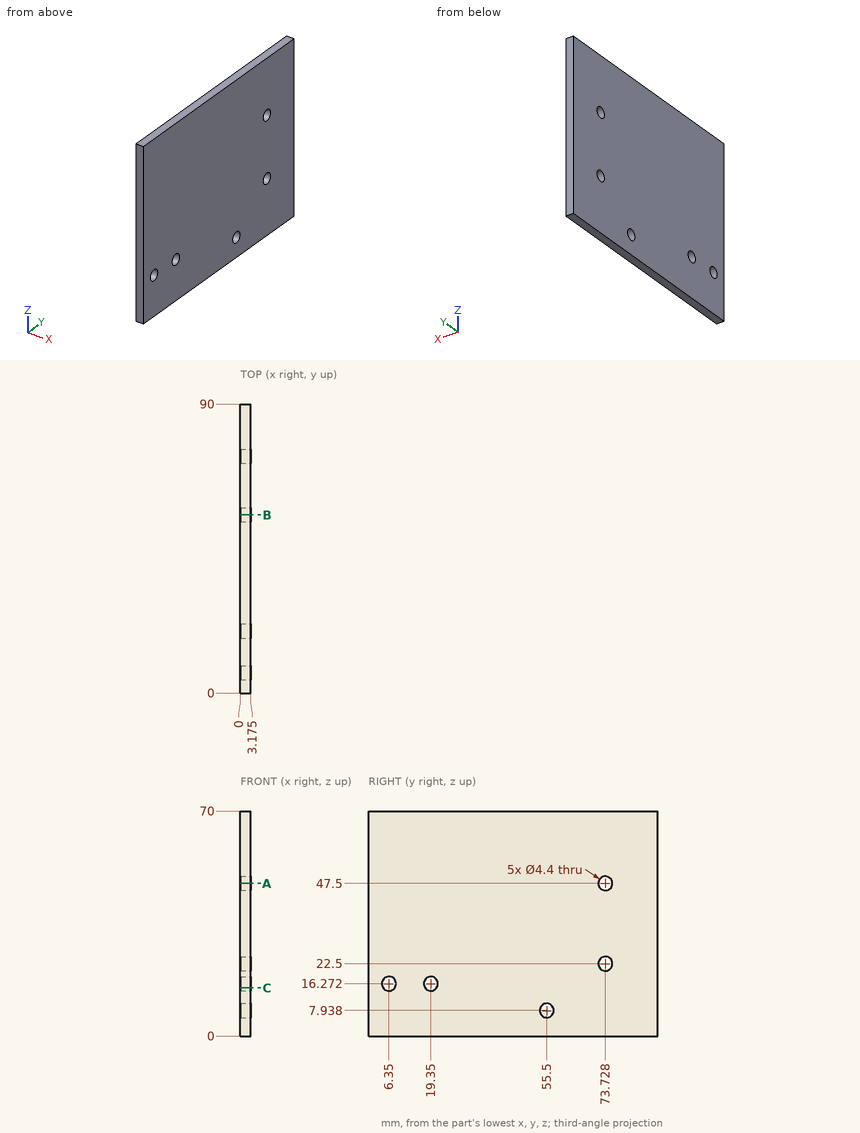
Geometry: see drawing. Coordinates: mm, zero at the bounding-box minimum. Coordinates: 2 decimals unless noted, no trailing zeros. Loops run counter-clockwise (first coordinate to the right, second up) from the corner with the lowest first, then second, coordinate; pieces in that order, holes last.
(1) Material intervals for probe 1 along Z at (x, y) = (1.7, 19.35); probe 2 along Y at (x, z) = (2.55, 46) (1 decimal); probe 3 along Y at (x, z) = (0.6, 23) (1 decimal), sorted ascending.
(2) Section B-B on y = 55.5. Return the cut outline in (x, z) (1 decimal).
(3) Section A-A on z = 47.5. Return the cut outline in (x, y) (1 decimal), then the cut area to 3 significant figures.
(4) First-contact query: pin 1 Ø2.5 at (y, z) = (73.728, 47.5) entering from -X; pin 2 Ø7 at (y, z) = (73.728, 22.5) entering from +X (1 decimal). Flat tips, straight axial feed; report the tip coordinate or a pass-through.
(5) Section C-C on z = 15. Return the cut outline in (x, y) (1 decimal).
Data:
1. probe 1: z = 0 to 14.07, 18.47 to 70
1. probe 2: y = 0 to 72.1, 75.3 to 90
1. probe 3: y = 0 to 71.6, 75.9 to 90
2. outline: (0, 0) - (3.2, 0) - (3.2, 5.7) - (0, 5.7) - close; (0, 10.1) - (3.2, 10.1) - (3.2, 70) - (0, 70) - close
3. outline: (0, 0) - (3.2, 0) - (3.2, 71.5) - (0, 71.5) - close; (0, 75.9) - (3.2, 75.9) - (3.2, 90) - (0, 90) - close
3. area: 272 mm2
4. pin 1: passes through
4. pin 2: stops at x = 3.2
5. outline: (0, 0) - (3.2, 0) - (3.2, 4.6) - (0, 4.6) - close; (0, 8.1) - (3.2, 8.1) - (3.2, 17.6) - (0, 17.6) - close; (0, 21.1) - (3.2, 21.1) - (3.2, 90) - (0, 90) - close
